Verification items for the finished model (mm, model axes). A direction names the side the tool comes from. Round coordinates to 2 decimals unless told otherwise and drop trailing zeros. Write each loop counter-clockwise with the first axis right and the second up, starting at its lowest first coordinate (ties: lowest second). Pieces come first, ordered by that corner, then holes. Notation, with made-up numbers: (-37, 77) - (11, 77) arc R31 cw to (11, 114) - close; hole circle Ø10 at (10.25, 21). An arc over 180 degrees is marked (long way). Answer as a JSON object with one key per item and string values.
```python
from build123d import *

# Parameters (mm, degrees)
SKETCH1_W           = 165.1
SKETCH1_H           = 203.2
BOSS_EXTRUDE1_DEPTH = 6.35
FILLET1_R           = 12.7
FILLET2_R           = 1.27


with BuildPart() as part:
    # Sketch1 → Boss-Extrude1 (new body)
    with BuildSketch(Plane(origin=(0, 0, 0), x_dir=(1, 0, 0), z_dir=(0, 1, 0))):
        Rectangle(SKETCH1_W, SKETCH1_H)
        with BuildLine():
            ThreePointArc((67.564, -50.8), (66.373681959, -53.673681959), (63.5, -54.864))
            Line((63.5, -54.864), (-63.5, -54.864))
            ThreePointArc((-63.5, -54.864), (-67.564, -50.8), (-63.5, -46.736))
            Line((-63.5, -46.736), (63.5, -46.736))
            ThreePointArc((63.5, -46.736), (66.373681959, -47.926318041), (67.564, -50.8))
        make_face(mode=Mode.SUBTRACT)
        with BuildLine():
            ThreePointArc((-63.5, 46.736), (-67.564, 50.8), (-63.5, 54.864))
            Line((-63.5, 54.864), (63.5, 54.864))
            ThreePointArc((63.5, 54.864), (66.373681959, 53.673681959), (67.564, 50.8))
            ThreePointArc((67.564, 50.8), (66.373681959, 47.926318041), (63.5, 46.736))
            Line((63.5, 46.736), (-63.5, 46.736))
        make_face(mode=Mode.SUBTRACT)
    extrude(amount=BOSS_EXTRUDE1_DEPTH)

    # Fillet1
    fillet1_edges = [part.edges().sort_by_distance(p)[0] for p in [
        (-82.55, 3.175, 101.6),
        (-82.55, 3.175, -101.6),
    ]]
    fillet(fillet1_edges, radius=FILLET1_R)

    # Fillet2
    fillet2_edges = [part.edges().sort_by_distance(p)[0] for p in [
        (82.55, 3.175, -101.6),
        (82.55, 3.175, 101.6),
    ]]
    fillet(fillet2_edges, radius=FILLET2_R)


solid = part.part
```
Q1. Section check B-B, the plane y = 3.75. Record the cut outline in (x, z).
Geometry check:
{"outline": "(-82.55, -88.9) arc R12.7 ccw to (-69.85, -101.6) - (81.28, -101.6) arc R1.27 ccw to (82.55, -100.33) - (82.55, 100.33) arc R1.27 ccw to (81.28, 101.6) - (-69.85, 101.6) arc R12.7 ccw to (-82.55, 88.9) - close; hole (-63.5, -54.86) - (63.5, -54.86) arc R4.06 ccw to (63.5, -46.74) - (-63.5, -46.74) arc R4.06 ccw to start; hole (-63.5, 46.74) - (63.5, 46.74) arc R4.06 ccw to (63.5, 54.86) - (-63.5, 54.86) arc R4.06 ccw to start"}
Q2. Material ranges on line 1 along Z through (x, y) = (-17.5, 0.5); line 2 along X through (y, z) = (3, -89.5); line 3 along X through (y, z) = (1.25, -49), recorded low to high. Write a range as [from, to].
Geometry check:
{"line 1": "z = [-101.6, -54.86], [-46.74, 46.74], [54.86, 101.6]", "line 2": "x = [-82.54, 82.55]", "line 3": "x = [-82.55, -67.14], [67.14, 82.55]"}
Q3. Section check A-A, the plane x = -37. Record the cut outline in (y, z).
Geometry check:
{"outline": "(0, -101.6) - (6.35, -101.6) - (6.35, -54.86) - (0, -54.86) - close; (0, -46.74) - (6.35, -46.74) - (6.35, 46.74) - (0, 46.74) - close; (0, 54.86) - (6.35, 54.86) - (6.35, 101.6) - (0, 101.6) - close"}
Q4. Release check for a two-part mould opening along Z. For faces 1 (the flat face through (5, 3, 101.6)), 2 (the flat face through (-1, 6.35, -1)), 3 (the flat face through (1, 3, 54.864)) record: released by +Z, released by -Z, zero draft, split by the parting line, or undercut.
Geometry check:
{"face 1": "released by +Z", "face 2": "zero draft", "face 3": "undercut"}
Q5. Set-up check for faces 4 (the cylindrical face through (-78.93, 3.22, -97.78)), 5 (the flat face through (1, 3, -46.736)): record each of +Z, -Z, +X, -X, +Y, -Y from which the full face is reachable in a straight line by a thin tool's end or side.
Geometry check:
{"face 4": "-Z, -X, +Y, -Y", "face 5": "+Y, -Y"}
